Here's the drawing with two shaded views (mm, measured from the low corner). I have some questions. Give positions to 0.01 mm unless a question says otherwise; leave off trailing zeros. Use a Markdown table: item, result. Add a question column.
1) Will these pins go through, and if not, where does the flat tip stop? pin 1 Ø1 at (y, z) = (17, 3) entering from +X; pin 2 Ø8 at (x, y) = (57, 18) entering from -Z; pin 3 Ø2 at (y, z) = (7, 3.5) entering from +X.
2) Suppose I cut it at A-A on z = 1.2. Count the separate pieces of the cut face and the enclosed holes in it, and give its area (3 significant figures).
3) If I drill on line 1 along X through (y, z) = (10.25, 1.75); line 2 along Y through (x, z) = (10, 3.8); line 3 along X through (y, z) = (6.25, 3.15), over which ranges is the centre line in solid material (lowest first)? Write a range as [from, to].
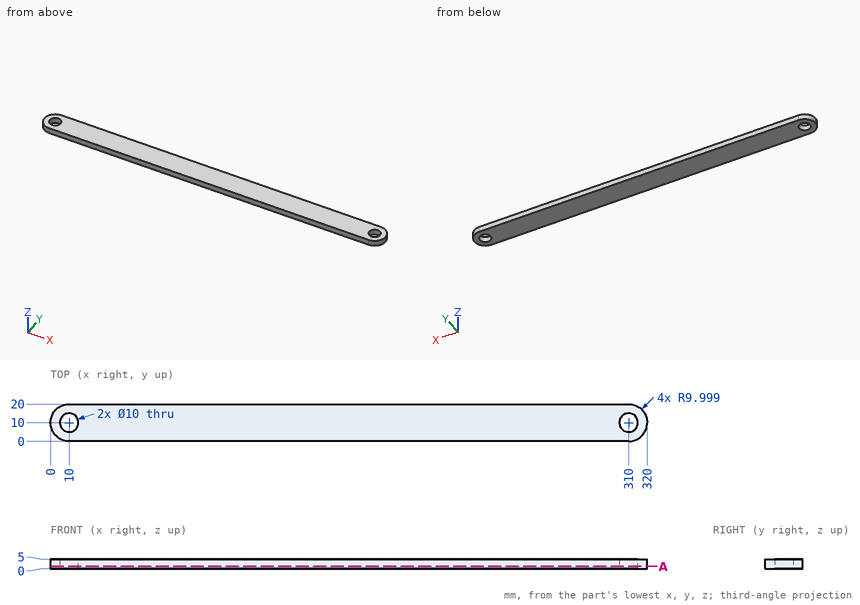
Answer block:
| question | item | result |
|---|---|---|
| 1 | pin 1 | stops at x = 317.6 |
| 1 | pin 2 | stops at z = 0 |
| 1 | pin 3 | stops at x = 319.8 |
| 2 | separate pieces | 1 |
| 2 | enclosed holes | 2 |
| 2 | area | 6,160 mm^2 |
| 3 | line 1 | x = [0, 5.01], [14.99, 305.01], [314.99, 320] |
| 3 | line 2 | y = [0, 5], [15, 20] |
| 3 | line 3 | x = [0.73, 6.69], [13.31, 306.69], [313.31, 319.27] |
